For this review, take the finished solid that the model builds, in its own axes (mm). A direction names the side the tool comes from. Round coordinates to 2 decimals unless told otherwise and drop trailing zeros. Write each loop counter-clockwise with the first axis right and the second up, starting at its lowest first coordinate (ties: lowest second). Pieces come first, ordered by that corner, then holes.
from build123d import *

# Parameters (mm, degrees)
BOSS_EXTRUDE1_DEPTH = 20
FILLET1_R           = 10
SKETCH2_R           = 2.5
CUT_EXTRUDE1_DEPTH  = 40
FILLET2_R           = 2
SKETCH3_R           = 2.5
CUT_EXTRUDE2_DEPTH  = 10


# Some blends are built 0.0001 mm under size
with BuildPart() as part:
    # Sketch1 → Boss-Extrude1 (new body)
    with BuildSketch(Plane(origin=(0, 0, 0), x_dir=(1, 0, 0), z_dir=(0, 1, 0))):
        with BuildLine():
            Line((27.849705815, 9.375), (27.849705815, 15))
            Line((27.849705815, 15), (42.849705815, 15))
            Line((42.849705815, 15), (42.849705815, 20))
            Line((42.849705815, 20), (27.849705815, 20))
            Line((27.849705815, 20), (-2.537743238, 14.78377013))
            ThreePointArc((-2.537743238, 14.78377013), (-15, 0), (-2.537743238, -14.78377013))
            Line((-2.537743238, -14.78377013), (15.176440556, -17.824540498))
            Line((15.176440556, -17.824540498), (6.327966589, -7.743180151))
            ThreePointArc((6.327966589, -7.743180151), (-6.707251498, 7.417059885), (7.069754095, -7.072381285))
            Line((7.069754095, -7.072381285), (16.743020962, -18.093455585))
            Line((16.743020962, -18.093455585), (27.849705815, -20))
            Line((27.849705815, -20), (42.849705815, -20))
            Line((42.849705815, -20), (42.849705815, -15))
            Line((42.849705815, -15), (27.849705815, -15))
            Line((27.849705815, -15), (27.849705815, -9.375))
            Line((27.849705815, -9.375), (42.849705815, -9.375))
            Line((42.849705815, -9.375), (42.849705815, -6.875))
            Line((42.849705815, -6.875), (27.849705815, -6.875))
            Line((27.849705815, -6.875), (27.849705815, -1.25))
            Line((27.849705815, -1.25), (42.849705815, -1.25))
            Line((42.849705815, -1.25), (42.849705815, 1.25))
            Line((42.849705815, 1.25), (27.849705815, 1.25))
            Line((27.849705815, 1.25), (27.849705815, 6.875))
            Line((27.849705815, 6.875), (42.849705815, 6.875))
            Line((42.849705815, 6.875), (42.849705815, 9.375))
            Line((42.849705815, 9.375), (27.849705815, 9.375))
        make_face()
    extrude(amount=BOSS_EXTRUDE1_DEPTH)

    # Fillet1
    fillet1_edges = [part.edges().sort_by_distance(p)[0] for p in [
        (42.849705815, 0, 17.5),
        (42.849705815, 0, 8.125),
        (42.849705815, 0, 0),
        (42.849705815, 0, -8.125),
        (42.849705815, 0, -17.5),
        (42.849705815, 20, -17.5),
        (42.849705815, 20, -8.125),
        (42.849705815, 20, 0),
        (42.849705815, 20, 8.125),
        (42.849705815, 20, 17.5),
    ]]
    fillet(fillet1_edges, radius=FILLET1_R - 0.0001)  # a hair under: the kernel refuses the full size

    # Sketch2 → Cut-Extrude1 (cut)
    with BuildSketch(Plane(origin=(0, 0, -20), x_dir=(-1, 0, 0), z_dir=(0, 0, -1))):
        with Locations((-35.349705815, 10)):
            Circle(SKETCH2_R)
    extrude(amount=-CUT_EXTRUDE1_DEPTH, mode=Mode.SUBTRACT)

    # Fillet2
    # the kernel refuses this fillet: 2 mm, written as the material it takes off along each edge
    with BuildSketch(Plane(origin=(39.676721919, 0, -22.03019459), x_dir=(0.16918288251037936, 0, 0.9855846753402162), z_dir=(-0.9855846753402161, 0, 0.16918288251037933))) as fillet2_piece_1:
        with BuildLine():
            CenterArc((FILLET2_R, FILLET2_R), FILLET2_R, 180, 90)
            Line((0, FILLET2_R), (-FILLET2_R * 0.02, FILLET2_R))
            Line((-FILLET2_R * 0.02, FILLET2_R), (-FILLET2_R * 0.02, -FILLET2_R * 0.02))
            Line((-FILLET2_R * 0.02, -FILLET2_R * 0.02), (FILLET2_R, -FILLET2_R * 0.02))
            Line((FILLET2_R, -FILLET2_R * 0.02), (FILLET2_R, 0))
        make_face()
    extrude(amount=42.831900914, mode=Mode.SUBTRACT)
    with BuildSketch(Plane(origin=(-2.537743238, 0, 14.78377013), x_dir=(0.16918288251037944, 0, -0.9855846753402161), z_dir=(0.9855846753402161, 0, 0.16918288251037944))) as fillet2_piece_2:
        with BuildLine():
            CenterArc((FILLET2_R, FILLET2_R), FILLET2_R, 180, 90)
            Line((0, FILLET2_R), (-FILLET2_R * 0.02, FILLET2_R))
            Line((-FILLET2_R * 0.02, FILLET2_R), (-FILLET2_R * 0.02, -FILLET2_R * 0.02))
            Line((-FILLET2_R * 0.02, -FILLET2_R * 0.02), (FILLET2_R, -FILLET2_R * 0.02))
            Line((FILLET2_R, -FILLET2_R * 0.02), (FILLET2_R, 0))
        make_face()
    extrude(amount=29.973274379, mode=Mode.SUBTRACT)
    with BuildSketch(Plane(origin=(39.676721919, 20, -22.03019459), x_dir=(0.16918288251037936, 0, 0.9855846753402162), z_dir=(-0.9855846753402161, 0, 0.16918288251037933))) as fillet2_piece_3:
        with BuildLine():
            CenterArc((FILLET2_R, -FILLET2_R), FILLET2_R, 90, 90)
            Line((0, -FILLET2_R), (-FILLET2_R * 0.02, -FILLET2_R))
            Line((-FILLET2_R * 0.02, -FILLET2_R), (-FILLET2_R * 0.02, FILLET2_R * 0.02))
            Line((-FILLET2_R * 0.02, FILLET2_R * 0.02), (FILLET2_R, FILLET2_R * 0.02))
            Line((FILLET2_R, FILLET2_R * 0.02), (FILLET2_R, 0))
        make_face()
    extrude(amount=42.831900914, mode=Mode.SUBTRACT)
    with BuildSketch(Plane(origin=(-2.537743238, 20, 14.78377013), x_dir=(0.16918288251037944, 0, -0.9855846753402161), z_dir=(0.9855846753402161, 0, 0.16918288251037944))) as fillet2_piece_4:
        with BuildLine():
            CenterArc((FILLET2_R, -FILLET2_R), FILLET2_R, 90, 90)
            Line((0, -FILLET2_R), (-FILLET2_R * 0.02, -FILLET2_R))
            Line((-FILLET2_R * 0.02, -FILLET2_R), (-FILLET2_R * 0.02, FILLET2_R * 0.02))
            Line((-FILLET2_R * 0.02, FILLET2_R * 0.02), (FILLET2_R, FILLET2_R * 0.02))
            Line((FILLET2_R, FILLET2_R * 0.02), (FILLET2_R, 0))
        make_face()
    extrude(amount=29.973274379, mode=Mode.SUBTRACT)
    with BuildSketch(Plane(origin=(4.916004858, 0, 16.063260995), x_dir=(0.16918288251037944, 0, -0.9855846753402161), z_dir=(0.9855846753402161, 0, 0.16918288251037944))) as fillet2_piece_5:
        with BuildLine():
            CenterArc((FILLET2_R, FILLET2_R), FILLET2_R, 180, 90)
            Line((0, FILLET2_R), (-FILLET2_R * 0.02, FILLET2_R))
            Line((-FILLET2_R * 0.02, FILLET2_R), (-FILLET2_R * 0.02, -FILLET2_R * 0.02))
            Line((-FILLET2_R * 0.02, -FILLET2_R * 0.02), (FILLET2_R, -FILLET2_R * 0.02))
            Line((FILLET2_R, -FILLET2_R * 0.02), (FILLET2_R, 0))
        make_face()
    extrude(amount=35.269133064, mode=Mode.SUBTRACT)
    with BuildSketch(Plane(origin=(4.916004858, 20, 16.063260995), x_dir=(0.16918288251037944, 0, -0.9855846753402161), z_dir=(0.9855846753402161, 0, 0.16918288251037944))) as fillet2_piece_6:
        with BuildLine():
            CenterArc((FILLET2_R, -FILLET2_R), FILLET2_R, 90, 90)
            Line((0, -FILLET2_R), (-FILLET2_R * 0.02, -FILLET2_R))
            Line((-FILLET2_R * 0.02, -FILLET2_R), (-FILLET2_R * 0.02, FILLET2_R * 0.02))
            Line((-FILLET2_R * 0.02, FILLET2_R * 0.02), (FILLET2_R, FILLET2_R * 0.02))
            Line((FILLET2_R, FILLET2_R * 0.02), (FILLET2_R, 0))
        make_face()
    extrude(amount=35.269133064, mode=Mode.SUBTRACT)
    with BuildSketch(Plane(origin=(0, 0, 0), x_dir=(-0.16918288251037905, 0, -0.9855846753402162), z_dir=(0.9855846753402162, 0, -0.16918288251037905))) as fillet2_piece_7:
        with BuildLine():
            CenterArc((15 - FILLET2_R, FILLET2_R), FILLET2_R, 270, 90)
            Line((15, FILLET2_R), (15 + FILLET2_R * 0.02, FILLET2_R))
            Line((15 + FILLET2_R * 0.02, FILLET2_R), (15 + FILLET2_R * 0.02, -FILLET2_R * 0.02))
            Line((15 + FILLET2_R * 0.02, -FILLET2_R * 0.02), (15 - FILLET2_R, -FILLET2_R * 0.02))
            Line((15 - FILLET2_R, -FILLET2_R * 0.02), (15 - FILLET2_R, 0))
        make_face()
    revolve(axis=Axis((0, 0, 0), (0, 1, 0)), revolution_arc=160.519372943, mode=Mode.SUBTRACT)
    with BuildSketch(Plane(origin=(0, 20, 0), x_dir=(-0.16918288251037905, 0, -0.9855846753402162), z_dir=(0.9855846753402162, 0, -0.16918288251037905))) as fillet2_piece_8:
        with BuildLine():
            CenterArc((15 - FILLET2_R, -FILLET2_R), FILLET2_R, 0, 90)
            Line((15, -FILLET2_R), (15 + FILLET2_R * 0.02, -FILLET2_R))
            Line((15 + FILLET2_R * 0.02, -FILLET2_R), (15 + FILLET2_R * 0.02, FILLET2_R * 0.02))
            Line((15 + FILLET2_R * 0.02, FILLET2_R * 0.02), (15 - FILLET2_R, FILLET2_R * 0.02))
            Line((15 - FILLET2_R, FILLET2_R * 0.02), (15 - FILLET2_R, 0))
        make_face()
    revolve(axis=Axis((0, 20, 0), (0, 1, 0)), revolution_arc=160.519372943, mode=Mode.SUBTRACT)

    # Sketch3 → Cut-Extrude2 (cut)
    with BuildSketch(Plane(origin=(-2.537743238, 0, 14.78377013), x_dir=(0.9855846753402161, 0, 0.16918288251037955), z_dir=(-0.16918288251037955, 0, 0.9855846753402161))):
        with Locations((12.973274379, 10)):
            Circle(SKETCH3_R)
    extrude(amount=-CUT_EXTRUDE2_DEPTH, mode=Mode.SUBTRACT)


solid = part.part
(1) Mouldability with a two-part tool opening along X and no side actions: class faces 1 (the face through (12.87, 9.89, -17.43)), 2 (the face through (40, 16.99, -8.14)), 3 (the face through (11.906, 10.035, 7.117)), 4 (the face through (33.6, 12.1, -15)) as pulls with the +X half, pulls with the -X half, needs draft (parallel to the pull), parting line crosses it, or undercut.
Geometry check:
face 1: pulls with the -X half
face 2: pulls with the +X half
face 3: undercut
face 4: needs draft
(2) We need section B-B, the plane y = 3.75. Give the boundary of the cut face in (x, z) (3 decimals), and give its area (3 significant figures).
Geometry check:
outline: (-2.538, -14.784) - (27.85, -20) - (40.656, -20) - (40.656, -15) - (27.85, -15) - (27.85, -9.375) - (40.656, -9.375) - (40.656, -6.875) - (27.85, -6.875) - (27.85, -1.25) - (40.656, -1.25) - (40.656, 1.25) - (27.85, 1.25) - (27.85, 6.875) - (40.656, 6.875) - (40.656, 9.375) - (27.85, 9.375) - (27.85, 15) - (40.656, 15) - (40.656, 20) - (27.85, 20) - (16.743, 18.093) - (7.07, 7.072) arc R10 cw (long way) to (6.328, 7.743) - (15.176, 17.825) - (-2.538, 14.784) arc R15 ccw to start
area: 1,230 mm2
(3) For pin 1 Ø4.5 at (y, z) = (12.5, -3) entering from +X; pin 2 Ø8 at (y, z) = (16.5, 13) entering from -X; pin 3 Ø6 at (y, z) = (14.5, 4.5) entering from +X, all flat-tipped, find the tip position at first contact; note any pin that passes through.
Geometry check:
pin 1: stops at x = 42.79
pin 2: stops at x = -12
pin 3: stops at x = 42.49
(4) We need section A-A, the plane z = 0. State how many separate pieces and enclosed holes the cut face has, and give its area (3 significant figures).
Geometry check:
separate pieces: 2
enclosed holes: 1
area: 693 mm2
(5) For line 1 along Z through (x, y) = (35, 12.75) (3 decimals); line 2 along X through (y, z) = (10.25, 9); line 3 along Z through (x, y) = (-6.5, 18.5), list the stretches that pass through material, from the lowest coordinate up.
Geometry check:
line 1: z = -20 to -15, -9.375 to -6.875, -1.25 to 1.25, 6.875 to 9.375, 15 to 20
line 2: x = -12 to -4.36, 4.36 to 7.43, 8.76 to 9.09, 14.14 to 32.86, 37.84 to 42.85
line 3: z = -13.45 to -7.6, 7.6 to 13.45
(6) We need section D-D, the plane y = 17.25. Give the boundary of the cut face in (x, z) (3 decimals).
Geometry check:
outline: (-2.538, -14.784) - (27.85, -20) - (39.737, -20) - (39.737, -15) - (27.85, -15) - (27.85, -9.375) - (39.737, -9.375) - (39.737, -6.875) - (27.85, -6.875) - (27.85, -1.25) - (39.737, -1.25) - (39.737, 1.25) - (27.85, 1.25) - (27.85, 6.875) - (39.737, 6.875) - (39.737, 9.375) - (27.85, 9.375) - (27.85, 15) - (39.737, 15) - (39.737, 20) - (27.85, 20) - (16.743, 18.093) - (7.07, 7.072) arc R10 cw (long way) to (6.328, 7.743) - (15.176, 17.825) - (-2.538, 14.784) arc R15 ccw to start
(7) For faces 5 (the face through (27.85, 10, -12)), 6 (the face through (9.8, 7.6, 11.7)), 7 (the face through (33.6, 12, 20)), list the 3-axis set-ups (+Z, -Z, +X, -X, +Y, -Y) from which the entire face can be reached by the end or side of a thin tool; tool diameter is ignored.
Geometry check:
face 5: +X, +Y, -Y
face 6: +Y, -Y
face 7: +Z, +X, -X, +Y, -Y
